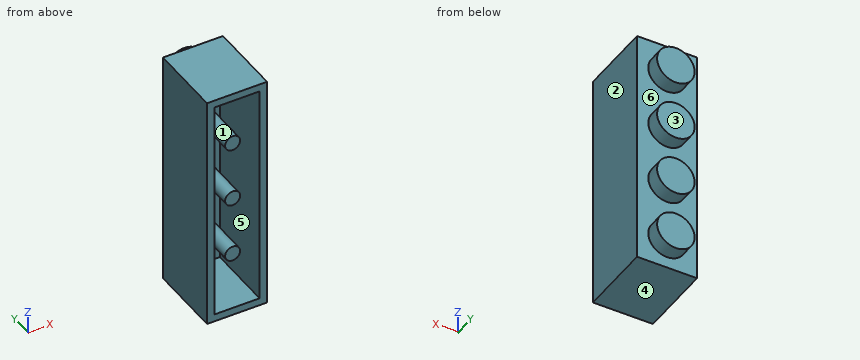
from build123d import *

# Parameters (mm, degrees)
SKETCH1_W                 = 8
SKETCH1_H                 = 32
BASE_EXTRUDE_DEPTH        = 5
SKETCH2_R                 = 2.5
BOSS_EXTRUDE1_DEPTH       = 2
TOP_BUTTON_PATTERN_COUNT  = 4
TOP_BUTTON_PATTERN_PITCH  = 8
SHELL1_T                  = -1
SKETCH3_R                 = 1
BOTTOM_POST_DEPTH         = 8
BOTTOM_POST_PATTERN_COUNT = 3
BOTTOM_POST_PATTERN_PITCH = 8


with BuildPart() as part:
    # Sketch1 → Base-Extrude (new, symmetric)
    with BuildSketch(Plane(origin=(0, 0, 0), x_dir=(1, 0, 0), z_dir=(0, 1, 0))):
        Rectangle(SKETCH1_W, SKETCH1_H)
    extrude(amount=BASE_EXTRUDE_DEPTH, both=True)

    # Sketch2 → Boss-Extrude1 (add)
    with BuildSketch(Plane(origin=(0, 5, 0), x_dir=(-1, 0, 0), z_dir=(0, 1, 0))):
        with Locations(Location((0, 12, 0), (0, 0, 90))):
            Circle(SKETCH2_R)
    boss_extrude1 = extrude(amount=BOSS_EXTRUDE1_DEPTH)

    # Top Button Pattern: Boss-Extrude1 ×4
    with Locations(*[(0, 0, -i * TOP_BUTTON_PATTERN_PITCH) for i in range(1, TOP_BUTTON_PATTERN_COUNT)]):
        add(boss_extrude1)

    # Shell1
    shell1_openings = [part.faces().sort_by_distance(p)[0] for p in [
        (0, -5, 0),
    ]]
    offset(amount=SHELL1_T, openings=shell1_openings, kind=Kind.INTERSECTION)

    # Sketch3 → Bottom Post (add)
    with BuildSketch(Plane.XZ.offset(-4)):
        with Locations(Location((0, 8, 0), (0, 0, 90))):
            Circle(SKETCH3_R)
    bottom_post = extrude(amount=BOTTOM_POST_DEPTH)

    # Bottom Post Pattern: Bottom Post ×3
    with Locations(*[(0, 0, -i * BOTTOM_POST_PATTERN_PITCH) for i in range(1, BOTTOM_POST_PATTERN_COUNT)]):
        add(bottom_post)


solid = part.part
Model file for the job. Use its own axes, mm. Face numbers are marked on the shaded views. A direction names the side the tool comes from. Give positions to 0.01 mm unless a question says otherwise; leave off trailing zeros. Loops run counter-clockwise (first coordinate to the right, second up) from the corner with the lowest first, then second, coordinate; pieces in that order, holes last.
1) Flat gauge pins, fed straight in: pin 1 Ø1.6 at (x, z) = (0.5, 0) entering from -Y; pin 2 Ø3 at (x, z) = (1, -5) entering from -Y; pin 3 Ø1.8 at (x, z) = (0, 4) entering from -Y. Where does each tip first touch, or does it go through?
2) Saw through at D-D (z = 0). Write the cut outline in (x, y).
3) Wall check: line 1 (Z direction, x = 0, y = 4.8); line 2 (X direction, y = -1.75, z = 0); line 3 (X direction, y = -3.25, z = -5). Give the ranges that are in metal, low to high.
4) Tool access for the marked faces 4, 5 and 6: list every direction of +Z, -Z, +X, -X, +Y, -Y with a clear straight run to the whole face (end or side of a thin tool).
5) Saw through at B-B (z = -4). Write the cut outline in (x, y), plus the area to 3 significant figures.
6) Saw through at C-C (x = 2). Write the cut outline in (y, z).
7) Saw through at A-A (y = 0). Write the cut outline in (x, z), plus the area to 3 significant figures.
8) Pull direction X, two halves, no side cores. Call the marked faces 1, 2 and 3: +X half, -X half, draft (parallel to the pull), parting line (faces both ways), or undercut.
Answer block:
1. pin 1: stops at y = -4
1. pin 2: stops at y = 4
1. pin 3: stops at y = 6
2. outline: (-4, -5) - (-3, -5) - (-3, 4) - (-1, 4) - (-1, -4) - (1, -4) - (1, 4) - (3, 4) - (3, -5) - (4, -5) - (4, 5) - (-4, 5) - close
3. line 1: z = -16 to -13.5, -10.5 to -5.5, -2.5 to 2.5, 5.5 to 10.5, 13.5 to 16
3. line 2: x = -4 to -3, -1 to 1, 3 to 4
3. line 3: x = -4 to -3, 3 to 4
4. face 4: -Z, +X, -X, +Y, -Y
4. face 5: -Y
4. face 6: +Y
5. outline: (-4, -5) - (-3, -5) - (-3, 4) - (-1.5, 4) - (-1.5, 6) - (1.5, 6) - (1.5, 4) - (3, 4) - (3, -5) - (4, -5) - (4, 5) - (2.5, 5) - (2.5, 7) - (-2.5, 7) - (-2.5, 5) - (-4, 5) - close
5. area: 30.0 mm2
6. outline: (-5, -16) - (5, -16) - (5, -13.5) - (7, -13.5) - (7, -10.5) - (5, -10.5) - (5, -5.5) - (7, -5.5) - (7, -2.5) - (5, -2.5) - (5, 2.5) - (7, 2.5) - (7, 5.5) - (5, 5.5) - (5, 10.5) - (7, 10.5) - (7, 13.5) - (5, 13.5) - (5, 16) - (-5, 16) - (-5, 15) - (4, 15) - (4, -15) - (-5, -15) - close
7. outline: (-4, -16) - (4, -16) - (4, 16) - (-4, 16) - close; circle Ø2 at (0, -8); circle Ø2 at (0, 0); circle Ø2 at (0, 8); hole (-3, -15) - (3, -15) - (3, 15) - (-3, 15) - close
7. area: 85.4 mm2
8. face 1: undercut
8. face 2: +X half
8. face 3: draft
